from build123d import *

# Parameters (mm, degrees)
SKETCH_1_R          = 1.5
EXTRUDE_1_DEPTH     = 5
EXTRUDE_1_2_DEPTH   = 5
EXTRUDE_1_3_DEPTH   = 5
SKETCH_2_W          = 13
SKETCH_2_H          = 10.5
EXTRUDE_6_DEPTH     = 2
SKETCH_1_6_R        = 2.1
CUT_EXTRUDE_2_DEPTH = 7
FILLET_1_SIZE       = 4
SKETCH_1_7_R        = 0.95
CUT_EXTRUDE_3_DEPTH = 6


with BuildPart() as part:
    # Sketch 1 → Extrude 1 (new body)
    with BuildSketch(Plane(origin=(0, 0, 0), x_dir=(1, 0, 0), z_dir=(0, 1, 0))):
        with Locations(Location((-5, 0, 0), (0, 0, 270))):
            Circle(SKETCH_1_R)
    extrude(amount=EXTRUDE_1_DEPTH)



with BuildPart() as body_2:
    # Sketch 1 → Extrude 1 2 (new body)
    with BuildSketch(Plane(origin=(0, 0, 0), x_dir=(1, 0, 0), z_dir=(0, 1, 0))):
        with Locations(Location((0, 5, 0), (0, 0, 270))):
            Circle(SKETCH_1_R)
    extrude(amount=EXTRUDE_1_2_DEPTH)


with BuildPart() as body_3:
    # Sketch 1 → Extrude 1 3 (new body)
    with BuildSketch(Plane(origin=(0, 0, 0), x_dir=(1, 0, 0), z_dir=(0, 1, 0))):
        with Locations(Location((5, 0, 0), (0, 0, 270))):
            Circle(SKETCH_1_R)
    extrude(amount=EXTRUDE_1_3_DEPTH)


with BuildPart() as part_1:
    add(part.part)

    add(body_2.part)  # Extrude 6 merges body 2

    add(body_3.part)  # Extrude 6 merges body 3
    # Sketch 2 → Extrude 6 (add)
    with BuildSketch(Plane(origin=(0, 5, 0), x_dir=(1, 0, 0), z_dir=(0, 1, 0))):
        with Locations((0, 1.25)):
            Rectangle(SKETCH_2_W, SKETCH_2_H)
    extrude(amount=EXTRUDE_6_DEPTH)

    # Sketch 1_6 → Cut-Extrude 2 (cut)
    with BuildSketch(Plane(origin=(0, 0, 0), x_dir=(1, 0, 0), z_dir=(0, 1, 0))):
        with Locations(Location((0, 0, 0), (0, 0, 90))):
            Circle(SKETCH_1_6_R)
    extrude(amount=CUT_EXTRUDE_2_DEPTH, mode=Mode.SUBTRACT)

    # Fillet 1
    # a fillet whose section is not a circle: 4 mm, written as the material it takes off along each edge
    with BuildSketch(Plane(origin=(6.5, -5, -6.5), x_dir=(-1, 0, 0), z_dir=(0, 1, 0)), Plane(origin=(6.5, -5, 4), x_dir=(0, 0, -1), z_dir=(0, 1, 0)), Plane(origin=(-6.5, -5, 4), x_dir=(1, 0, 0), z_dir=(0, 1, 0))) as fillet_1_piece_1:
        with BuildLine():
            add(Edge.make_bspline([(FILLET_1_SIZE, 0), (FILLET_1_SIZE * 0.831801948466, 0), (FILLET_1_SIZE * 0.663603896932, 0), (FILLET_1_SIZE * 0.292893218813, FILLET_1_SIZE * 0.0716919198361), (FILLET_1_SIZE * 0.0716919198361, FILLET_1_SIZE * 0.292893218813), (0, FILLET_1_SIZE * 0.663603896932), (0, FILLET_1_SIZE * 0.831801948466), (0, FILLET_1_SIZE)], knots=[0, 0, 0, 0, 0, 0, 0.5, 0.5, 1, 1, 1, 1, 1, 1], degree=5))
            Line((0, FILLET_1_SIZE), (0, 0))
            Line((0, 0), (FILLET_1_SIZE, 0))
        make_face()
    extrude(amount=22, mode=Mode.SUBTRACT)
    with BuildSketch(Plane(origin=(-6.5, -5, -6.5), x_dir=(1, 0, 0), z_dir=(0, 1, 0))) as fillet_1_piece_2:
        with BuildLine():
            add(Edge.make_bspline([(FILLET_1_SIZE, 0), (FILLET_1_SIZE * 0.831801948466, 0), (FILLET_1_SIZE * 0.663603896932, 0), (FILLET_1_SIZE * 0.292893218813, -FILLET_1_SIZE * 0.0716919198361), (FILLET_1_SIZE * 0.0716919198361, -FILLET_1_SIZE * 0.292893218813), (0, -FILLET_1_SIZE * 0.663603896932), (0, -FILLET_1_SIZE * 0.831801948466), (0, -FILLET_1_SIZE)], knots=[0, 0, 0, 0, 0, 0, 0.5, 0.5, 1, 1, 1, 1, 1, 1], degree=5))
            Line((0, -FILLET_1_SIZE), (0, 0))
            Line((0, 0), (FILLET_1_SIZE, 0))
        make_face()
    extrude(amount=22, mode=Mode.SUBTRACT)

    # Sketch 1_7 → Cut-Extrude 3 (cut)
    with BuildSketch(Plane(origin=(0, 0, 0), x_dir=(1, 0, 0), z_dir=(0, 1, 0))):
        with Locations(Location((5, 0, 0), (0, 0, 270))):
            Circle(SKETCH_1_7_R)
        with Locations(Location((0, 5, 0), (0, 0, 270))):
            Circle(SKETCH_1_7_R)
        with Locations(Location((-5, 0, 0), (0, 0, 270))):
            Circle(SKETCH_1_7_R)
    extrude(amount=CUT_EXTRUDE_3_DEPTH, mode=Mode.SUBTRACT)


solid = part_1.part
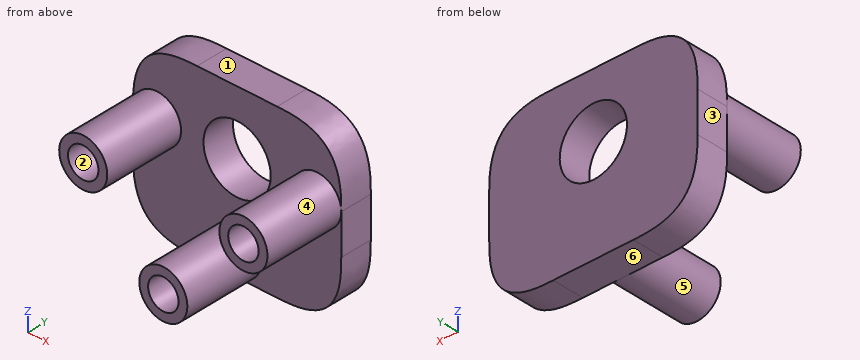
Verification items for the finished model (mm, model axes). Face numbers are marked on the shaded views. A direction names the side the tool comes from. Coordinates: 2 decimals unless noted, no trailing zeros. Order: outer loops, then holes, each group sorted by start corner. A loop starts at its lowest first (then second) coordinate and runs counter-clockwise, first axis right, second up. Notation, with made-up numbers: M -34,80.25 L 6,80.25 A8 cw 6,88.25 Z; hole C 43,28.5 d9. An arc over 180 degrees is marked long. One line per item, written item: value. Start each with the question number.
Item 1: Sectioned sample at A-A (y = 4.25). Enter the section's corners in (x, z).
Item 2: Access from +Z, -Z, +X, -X, +Y, -Y to the whole of each face (thin tool, end or side, straight path). Record for the marked faces 1 and 2.
Item 3: Sectioned sample at B-B (z = -1.75). Enter the section's corners in (x, y), then the cut area to 3 significant figures.
Item 4: Scan lines: probe 1 along X at (y, z) = (1.8, 0); probe 2 along X at (y, z) = (2.25, -5); probe 3 along X at (y, z) = (6.1, 0). Record each from-to range of solid material in increasing order.
Item 5: Gauge pin test, flat ends, axial feed: pin 1 (5.5 mm diameter, centred on x = 0, z = 0, fed in from -Y); pin 2 (1.5 mm diameter, centred on x = -5, z = 0, fed in from -Y); pin 3 (1.5 mm diameter, centred on y = 2.5, z = -3, fed in from -X). Record the tip position at first contact, or that the pin passes through.
Item 6: Mould release check, pull along X, two halves, no side actions. Record for the marked faces 3, 4, 5 and 6: released by +X, released by -X, zero draft, split by the parting line, or undercut.
Item 7: Sectioned sample at C-C (x = 1.75). Enter the section's corners in (y, z).
Conclusion:
1. outline: C -5,0 d3; C 0,-5 d3; C 5,0 d3; hole C -5,0 d1.9; hole C 0,-5 d1.9; hole C 5,0 d1.9
2. face 1: +Z, +X, -X, +Y, -Y
2. face 2: -Y
3. outline: M -6.5,5 L -1.16,5 L -1.16,7 L -6.5,7 Z; M 1.16,5 L 6.5,5 L 6.5,7 L 1.16,7 Z
3. area: 21.4 mm^2
4. probe 1: x = -6.5 to -5.95, -4.05 to -3.5, 3.5 to 4.05, 5.95 to 6.5
4. probe 2: x = -1.5 to -0.95, 0.95 to 1.5
4. probe 3: x = -6.5 to -2.1, 2.1 to 6.5
5. pin 1: stops at y = 5
5. pin 2: stops at y = 6
5. pin 3: stops at x = -0.83
6. face 3: released by -X
6. face 4: undercut
6. face 5: split by the parting line
6. face 6: zero draft
7. outline: M 5,-6.5 L 7,-6.5 L 7,-1.16 L 5,-1.16 Z; M 5,1.16 L 7,1.16 L 7,4 L 5,4 Z
